Verification items for this drawing (mm, ordinates from the low corner). A direction names the side the tool comes from. Coordinates: 2 decimals unless noted, no trailing zeros. Write each loop counter-clockwise with the first axis right and the second up, starting at its lowest first coordinate (ties: lowest second). Pieces come first, ordered by that corner, then holes. Notation, with made-up numbers: M 75,51.25 L 132,51.25 A14 cw 132,67.25 Z; hole C -35,33.5 d4. An arc over 180 degrees is marked long. Answer as CSV lines item,"result". Start each with the question number.
1) Go/stop test with flat-tipped pins: pin 1 Ø2 at (y, z) = (6.5, 12.5) entering from +X; pin 2 Ø6 at (x, z) = (9, 12) entering from +Y. Record where each tip stops, or that it passes through.
2) Material ranges on L1, parallel to Z at x = 13.25, y = 12.25; L2, parallel to Y at x = 8, z = 5.25; L3, parallel to X at y = 8, z = 9.25, recorded low to high. Write a range as [from, to].
3) Draft check along Z on the marked faces 3, 4 and 5. Enter one of: +Z half, -Z half, draft (parallel to the pull), parting line (faces both ways), or undercut.
4) Section check A-A (x = 8). Record the cut outline in (y, z), and give its area (3 significant figures).
5) Section check D-D (x = 1.25). Record the cut outline in (y, z).
6) Access from +Z, -Z, +X, -X, +Y, -Y to the whole of each face (thin tool, end or side, straight path). Record for the marked faces 1 and 2.
7) Section check C-C (z = 7.5). Record the cut outline in (x, y), and give its area (3 significant figures).
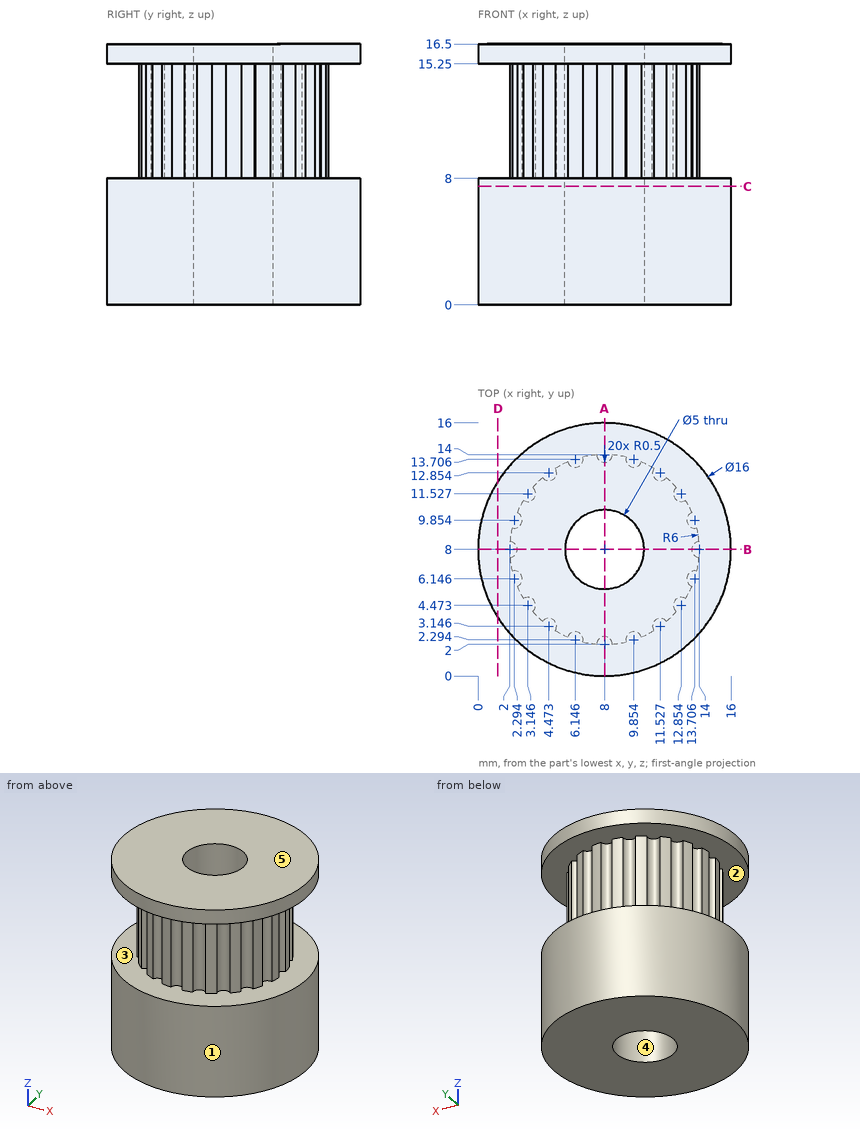
Results found:
1,pin 1,"stops at x = 13.98"
1,pin 2,"stops at y = 13.98"
2,L1,"z = [0, 8], [15.25, 16.5]"
2,L2,"y = [0, 5.5], [10.5, 16]"
2,L3,"x = [2.5, 5.5], [10.5, 13.5]"
3,face 3,"undercut"
3,face 4,"draft"
3,face 5,"+Z half"
4,outline,"M 0,0 L 5.5,0 L 5.5,16.5 L 0,16.5 L 0,15.25 L 2.5,15.25 L 2.5,8 L 0,8 Z; M 10.5,0 L 16,0 L 16,8 L 13.5,8 L 13.5,15.25 L 16,15.25 L 16,16.5 L 10.5,16.5 Z"
4,area,"145 mm2"
5,outline,"M 3.71,0 L 12.29,0 L 12.29,8 L 3.71,8 Z; M 3.71,15.25 L 12.29,15.25 L 12.29,16.5 L 3.71,16.5 Z"
6,face 1,"+Z, -Z"
6,face 2,"none"
7,outline,"C 8,8 d16; hole C 8,8 d5"
7,area,"181 mm2"
